Geometry: final body of the model. Coordinates: model frame, mm. Face numbers are marked on the shaded views. A direction names the side the tool comes from. Coordinates: 2 decimals unless noted, no trailing zeros. Loops run counter-clockwise (first coordinate to the right, second up) from the corner with the lowest first, then second, coordinate; pieces in that order, holes last. Notation, with made-up numbers: (41.5, -7) - (82.5, -7) arc R18 ccw to (82.5, 17) - close; hole circle Ø11 at (53.25, 39). An arc over 180 degrees is marked (long way). Put each result on its own line as item: value. Start each with the question number.
1) Material intervals for line 1 along Z through (x, y) = (4, 1.95); line 2 along Z through (x, y) = (83, -31); line 3 along Y through (x, z) = (119, -2.5), sorted ascending. Write a range as from..to.
2) Section A-A on x = -29.5. Output: boundary loops of the cut face in (y, z), and give its area (3 significant figures).
3) Contact query for flat-ended pins moving along their axis: pin 1 Ø4 at (x, z) = (-100, 17.1) entering from -Y; pin 2 Ø16.5 at (x, z) = (126, 13) entering from -Y; pin 3 Ø2 at (y, z) = (10, 49) entering from +X. Output: stop coordinate, or through.
4) Reachability of the marked faces 1 and 2 from +Z, -Z, +X, -X, +Y, -Y: full face, straight path, thin tool, end or side. Return the list, or none.
5) Section D-D on y = -64.5. Output: boundary loops of the cut face in (x, z), and give its area (3 significant figures).
6) Section B-B on x = 122.05. Count the separate pieces of the cut face and the enclosed holes in it, and give its area (3 significant figures).
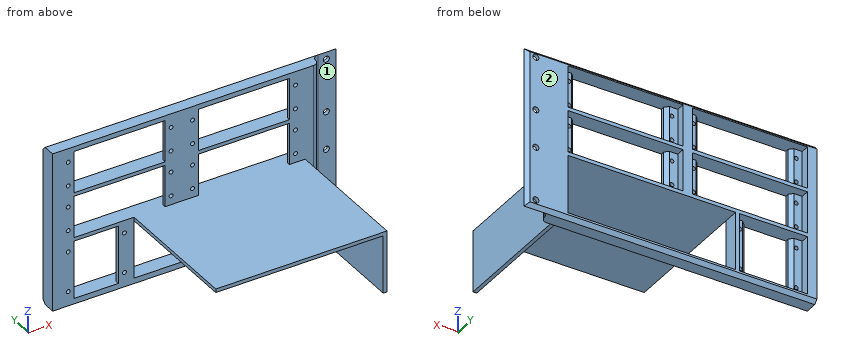
```python
from build123d import *

# Parameters (mm, degrees)
SKETCH1_W                      = 243
SKETCH1_H                      = 133.2
BOSS_EXTRUDE1_DEPTH            = 13
SKETCH32_W                     = 20
SKETCH32_H                     = 133.2
CUT_EXTRUDE10_DEPTH            = 10
FILLET1_START                  = -68
FILLET1_DEPTH                  = 136
FILLET1_START_2                = -66.6
FILLET1_2_DEPTH                = 133.2
M6X1_0_TAPPED_HOLE1_D          = 5
M6X1_0_TAPPED_HOLE1_DEPTH      = 15
M6X1_0_TAPPED_HOLE1_TIP        = 1.502151548
SKETCH36_W                     = 96
SKETCH36_H                     = 35
CUT_EXTRUDE11_DEPTH            = 7
SKETCH37_W                     = 76
SKETCH37_H                     = 35
CUT_EXTRUDE12_DEPTH            = 147.644331633
M4X0_7_TAPPED_HOLE1_AT_2_COUNT = 2
M4X0_7_TAPPED_HOLE1_AT_2_PITCH = 20
M4X0_7_TAPPED_HOLE1_AT_3_COUNT = 2
M4X0_7_TAPPED_HOLE1_AT_3_PITCH = 86
M4X0_7_TAPPED_HOLE1_AT_4_COUNT = 2
M4X0_7_TAPPED_HOLE1_AT_4_PITCH = 88.294960219
LPATTERN1_COUNT                = 2
LPATTERN1_PITCH                = 38
LPATTERN1_COUNT_DIR2           = 2
LPATTERN1_PITCH_DIR2           = 104
CHAMFER1_SIZE                  = 3
SKETCH41_W                     = 140
SKETCH41_H                     = 48.6
CUT_EXTRUDE13_DEPTH            = 30
BOSS_EXTRUDE2_DEPTH            = 110
SKETCH43_W                     = 57
SKETCH43_H                     = 48.6
CUT_EXTRUDE14_DEPTH            = 7
SKETCH44_W                     = 37
SKETCH44_H                     = 48.6
CUT_EXTRUDE15_DEPTH            = 17
CHAMFER2_SIZE                  = 3
M4X0_7_TAPPED_HOLE2_D          = 3.3
M4X0_7_TAPPED_HOLE2_DEPTH      = 10.1
M4X0_7_TAPPED_HOLE2_TIP        = 0.991420021


with BuildPart() as part:
    # Sketch1 → Boss-Extrude1 (new body)
    with BuildSketch(Plane(origin=(0, 0, 0), x_dir=(1, 0, 0), z_dir=(0, 1, 0))):
        with Locations((8.5, 0)):
            Rectangle(SKETCH1_W, SKETCH1_H)
    extrude(amount=BOSS_EXTRUDE1_DEPTH)

    # Sketch32 → Cut-Extrude10 (cut)
    with BuildSketch(Plane.XZ):
        with Locations((120, 0)):
            Rectangle(SKETCH32_W, SKETCH32_H)
    extrude(amount=-CUT_EXTRUDE10_DEPTH, mode=Mode.SUBTRACT)

    # Fillet1: read off the stored shape, not the designer's step
    # Fillet1 outline → Fillet1 (cut)
    with BuildSketch(Plane.XY.offset(FILLET1_START)):
        with BuildLine():
            Line((110, 0), (110, 5))
            ThreePointArc((110, 5), (108.535533906, 1.464466094), (105, 0))
            Line((105, 0), (110, 0))
        make_face()
    extrude(amount=FILLET1_DEPTH, mode=Mode.SUBTRACT)

    # Fillet1 2 outline → Fillet1 2 (add)
    with BuildSketch(Plane.XY.offset(FILLET1_START_2)):
        with BuildLine():
            ThreePointArc((110, 5), (111.464466094, 8.535533906), (115, 10))
            Line((115, 10), (110, 10))
            Line((110, 10), (110, 5))
        make_face()
    extrude(amount=FILLET1_2_DEPTH)

    # M6x1.0 Tapped Hole1
    with Locations(Plane(origin=(0, 13, 0), x_dir=(1, 0, 0), z_dir=(0, 1, 0))):
        with Locations((122.05, 60.25), (122.05, 15.75), (122.05, -16.05), (122.05, -60.55)):
            Hole(M6X1_0_TAPPED_HOLE1_D / 2, depth=M6X1_0_TAPPED_HOLE1_DEPTH)
            with Locations((0, 0, -(M6X1_0_TAPPED_HOLE1_DEPTH + M6X1_0_TAPPED_HOLE1_TIP / 2))):  # 118° drill point
                Cone(0, M6X1_0_TAPPED_HOLE1_D / 2, M6X1_0_TAPPED_HOLE1_TIP, mode=Mode.SUBTRACT)

    # Sketch36 → Cut-Extrude11 (cut)
    with BuildSketch(Plane(origin=(0, 13, 0), x_dir=(1, 0, 0), z_dir=(0, 1, 0))):
        with Locations((-57, -45.1)):
            Rectangle(SKETCH36_W, SKETCH36_H)
        with Locations((-57, -7.1)):
            Rectangle(SKETCH36_W, SKETCH36_H)
        with Locations((47, -7.1)):
            Rectangle(SKETCH36_W, SKETCH36_H)
        with Locations((47, -45.1)):
            Rectangle(SKETCH36_W, SKETCH36_H)
    extrude(amount=-CUT_EXTRUDE11_DEPTH, mode=Mode.SUBTRACT)

    # Sketch37 → Cut-Extrude12 (cut, through all)
    with BuildSketch(Plane(origin=(0, 13, 0), x_dir=(1, 0, 0), z_dir=(0, 1, 0))):
        with Locations((-57, -45.1)):
            Rectangle(SKETCH37_W, SKETCH37_H)
        with Locations((-57, -7.1)):
            Rectangle(SKETCH37_W, SKETCH37_H)
        with Locations((47, -7.1)):
            Rectangle(SKETCH37_W, SKETCH37_H)
        with Locations((47, -45.1)):
            Rectangle(SKETCH37_W, SKETCH37_H)
    extrude(amount=-CUT_EXTRUDE12_DEPTH, mode=Mode.SUBTRACT)

    # Sketch39 → M4x0.7 Tapped Hole1 (revolve, cut)
    with BuildSketch(Plane(origin=(-100, 6, 55.1), x_dir=(0, 0, 1), z_dir=(1, 0, 0))):
        Polygon((0, 0), (0, 11.091420021), (1.65, 10.1), (1.65, 0), align=None)
    m4x0_7_tapped_hole1 = revolve(axis=Axis((-100, 12.35, 55.1), (0, -1, 0)), mode=Mode.SUBTRACT)

    # M4x0.7 Tapped Hole1 at 2: M4x0.7 Tapped Hole1 ×2
    with Locations(*[(0, 0, -i * M4X0_7_TAPPED_HOLE1_AT_2_PITCH) for i in range(1, M4X0_7_TAPPED_HOLE1_AT_2_COUNT)]):
        add(m4x0_7_tapped_hole1, mode=Mode.SUBTRACT)

    # M4x0.7 Tapped Hole1 at 3: M4x0.7 Tapped Hole1 ×2
    with Locations(*[(i * M4X0_7_TAPPED_HOLE1_AT_3_PITCH, 0, 0) for i in range(1, M4X0_7_TAPPED_HOLE1_AT_3_COUNT)]):
        add(m4x0_7_tapped_hole1, mode=Mode.SUBTRACT)

    # M4x0.7 Tapped Hole1 at 4: M4x0.7 Tapped Hole1 ×2
    with Locations(*[Vector(0.9740080270391964, 0, -0.2265134946602783) * (i * M4X0_7_TAPPED_HOLE1_AT_4_PITCH) for i in range(1, M4X0_7_TAPPED_HOLE1_AT_4_COUNT)]):
        add(m4x0_7_tapped_hole1, mode=Mode.SUBTRACT)

    # LPattern1: M4x0.7 Tapped Hole1 2 × 2
    with Locations(*[(j * LPATTERN1_PITCH_DIR2, 0, -i * LPATTERN1_PITCH) for i in range(LPATTERN1_COUNT) for j in range(LPATTERN1_COUNT_DIR2) if (i, j) != (0, 0)]):
        add(m4x0_7_tapped_hole1, mode=Mode.SUBTRACT)

    # LPattern1 copy 1 sketch → LPattern1 copy 1 (revolve, cut)
    with BuildSketch(Plane(origin=(4, 6, 35.1), x_dir=(0, 0, 1), z_dir=(1, 0, 0))):
        Polygon((0, 0), (0, 11.091420021), (1.65, 10.1), (1.65, 0), align=None)
    revolve(axis=Axis((4, 12.35, 35.1), (0, -1, 0)), mode=Mode.SUBTRACT)

    # LPattern1 copy 2 sketch → LPattern1 copy 2 (revolve, cut)
    with BuildSketch(Plane(origin=(-100, 6, -2.9), x_dir=(0, 0, 1), z_dir=(1, 0, 0))):
        Polygon((0, 0), (0, 11.091420021), (1.65, 10.1), (1.65, 0), align=None)
    revolve(axis=Axis((-100, 12.35, -2.9), (0, -1, 0)), mode=Mode.SUBTRACT)

    # LPattern1 copy 3 sketch → LPattern1 copy 3 (revolve, cut)
    with BuildSketch(Plane(origin=(4, 6, -2.9), x_dir=(0, 0, 1), z_dir=(1, 0, 0))):
        Polygon((0, 0), (0, 11.091420021), (1.65, 10.1), (1.65, 0), align=None)
    revolve(axis=Axis((4, 12.35, -2.9), (0, -1, 0)), mode=Mode.SUBTRACT)

    # LPattern1 copy 4 sketch → LPattern1 copy 4 (revolve, cut)
    with BuildSketch(Plane(origin=(90, 6, 55.1), x_dir=(0, 0, 1), z_dir=(1, 0, 0))):
        Polygon((0, 0), (0, 11.091420021), (1.65, 10.1), (1.65, 0), align=None)
    revolve(axis=Axis((90, 12.35, 55.1), (0, -1, 0)), mode=Mode.SUBTRACT)

    # LPattern1 copy 5 sketch → LPattern1 copy 5 (revolve, cut)
    with BuildSketch(Plane(origin=(-14, 6, 17.1), x_dir=(0, 0, 1), z_dir=(1, 0, 0))):
        Polygon((0, 0), (0, 11.091420021), (1.65, 10.1), (1.65, 0), align=None)
    revolve(axis=Axis((-14, 12.35, 17.1), (0, -1, 0)), mode=Mode.SUBTRACT)

    # LPattern1 copy 6 sketch → LPattern1 copy 6 (revolve, cut)
    with BuildSketch(Plane(origin=(90, 6, 17.1), x_dir=(0, 0, 1), z_dir=(1, 0, 0))):
        Polygon((0, 0), (0, 11.091420021), (1.65, 10.1), (1.65, 0), align=None)
    revolve(axis=Axis((90, 12.35, 17.1), (0, -1, 0)), mode=Mode.SUBTRACT)

    # LPattern1 copy 7 sketch → LPattern1 copy 7 (revolve, cut)
    with BuildSketch(Plane(origin=(90, 6, 35.1), x_dir=(0, 0, 1), z_dir=(1, 0, 0))):
        Polygon((0, 0), (0, 11.091420021), (1.65, 10.1), (1.65, 0), align=None)
    revolve(axis=Axis((90, 12.35, 35.1), (0, -1, 0)), mode=Mode.SUBTRACT)

    # LPattern1 copy 8 sketch → LPattern1 copy 8 (revolve, cut)
    with BuildSketch(Plane(origin=(-14, 6, -2.9), x_dir=(0, 0, 1), z_dir=(1, 0, 0))):
        Polygon((0, 0), (0, 11.091420021), (1.65, 10.1), (1.65, 0), align=None)
    revolve(axis=Axis((-14, 12.35, -2.9), (0, -1, 0)), mode=Mode.SUBTRACT)

    # LPattern1 copy 9 sketch → LPattern1 copy 9 (revolve, cut)
    with BuildSketch(Plane(origin=(90, 6, -2.9), x_dir=(0, 0, 1), z_dir=(1, 0, 0))):
        Polygon((0, 0), (0, 11.091420021), (1.65, 10.1), (1.65, 0), align=None)
    revolve(axis=Axis((90, 12.35, -2.9), (0, -1, 0)), mode=Mode.SUBTRACT)

    # Chamfer1
    chamfer1_edges = [part.edges().sort_by_distance(p)[0] for p in [
        (-95, 6, 7.1),
        (-19, 6, 7.1),
        (-19, 6, 45.1),
        (-95, 6, 45.1),
        (85, 6, 7.1),
        (9, 6, 7.1),
        (9, 6, 45.1),
        (85, 6, 45.1),
        (8.5, 13, -66.6),
        (130, 13, 0),
        (8.5, 13, 66.6),
    ]]
    chamfer(chamfer1_edges, length=CHAMFER1_SIZE - 0.0001)  # a hair under: the kernel refuses the full size

    # Sketch41 → Cut-Extrude13 (cut)
    with BuildSketch(Plane(origin=(0, 13, 0), x_dir=(1, 0, 0), z_dir=(0, 1, 0))):
        with Locations((25, 37.7)):
            Rectangle(SKETCH41_W, SKETCH41_H)
    extrude(amount=-CUT_EXTRUDE13_DEPTH, mode=Mode.SUBTRACT)

    # Sketch42 → Boss-Extrude2 (add)
    with BuildSketch(Plane.XZ):
        Polygon((-45, -13.4), (95, -13.4), (95, -62), (98.143065291, -62), (98.143065291, -10.4), (95, -10.4), (-45, -10.4), align=None)
    extrude(amount=BOSS_EXTRUDE2_DEPTH)

    # Sketch43 → Cut-Extrude14 (cut)
    with BuildSketch(Plane(origin=(0, 13, 0), x_dir=(1, 0, 0), z_dir=(0, 1, 0))):
        with Locations((-76.5, 37.7)):
            Rectangle(SKETCH43_W, SKETCH43_H)
    extrude(amount=-CUT_EXTRUDE14_DEPTH, mode=Mode.SUBTRACT)

    # Sketch44 → Cut-Extrude15 (cut)
    with BuildSketch(Plane(origin=(0, 6, 0), x_dir=(1, 0, 0), z_dir=(0, 1, 0))):
        with Locations((-76.5, 37.7)):
            Rectangle(SKETCH44_W, SKETCH44_H)
    extrude(amount=-CUT_EXTRUDE15_DEPTH, mode=Mode.SUBTRACT)

    # Chamfer2
    chamfer2_edges = [part.edges().sort_by_distance(p)[0] for p in [
        (-95, 6, -37.7),
        (-58, 6, -37.7),
    ]]
    chamfer(chamfer2_edges, length=CHAMFER2_SIZE)

    # M4x0.7 Tapped Hole2
    with Locations(Plane(origin=(0, 6, 0), x_dir=(1, 0, 0), z_dir=(0, 1, 0))):
        with Locations((-100, 20.9), (-100, 54.5), (-53, 54.5), (-53, 20.9)):
            Hole(M4X0_7_TAPPED_HOLE2_D / 2, depth=M4X0_7_TAPPED_HOLE2_DEPTH)
            with Locations((0, 0, -(M4X0_7_TAPPED_HOLE2_DEPTH + M4X0_7_TAPPED_HOLE2_TIP / 2))):  # 118° drill point
                Cone(0, M4X0_7_TAPPED_HOLE2_D / 2, M4X0_7_TAPPED_HOLE2_TIP, mode=Mode.SUBTRACT)


solid = part.part
```
Answer block:
1. line 1: z = -66.6..-62, -13.4..-4.55, -1.25..15.45, 18.75..33.45, 36.75..53.45, 56.75..66.6
1. line 2: z = -13.4..-10.4
1. line 3: y = 10..13
2. outline: (-110, -13.4) - (13, -13.4) - (13, -10.4) - (-110, -10.4) - close; (0, -66.6) - (10, -66.6) - (13, -63.6) - (13, -62) - (0, -62) - close; (0, 24.6) - (13, 24.6) - (13, 27.6) - (0, 27.6) - close; (0, 62.6) - (13, 62.6) - (13, 63.6) - (10, 66.6) - (0, 66.6) - close
2. area: 511 mm²
3. pin 1: stops at y = 0
3. pin 2: stops at y = 10
3. pin 3: stops at x = 130
4. face 1: +Z, -Z, +X, -Y
4. face 2: +Z, -Z, +X, -X, +Y
5. outline: (-45, -13.4) - (95, -13.4) - (95, -62) - (98.14, -62) - (98.14, -10.4) - (-45, -10.4) - close
5. area: 582 mm²
6. separate pieces: 5
6. enclosed holes: 0
6. area: 331 mm²
